Part model, mm, in its own coordinate system. Give positions to 0.01 mm unless a question says otherwise; leave off trailing zeros. Order: outer loops, then holes, each group sorted by start corner. A loop starts at its lowest first (then second) coordinate and runs counter-clockwise, first axis right, second up. Notation, with made-up numbers: (23.25, -37) - (79.25, -37) arc R13 ccw to (79.25, -25) - close; hole circle Ø10 at (84.5, -34.75). An arc over 180 degrees is marked (long way). One line per item, written item: value.
```python
from build123d import *

# Parameters (mm, degrees)
SKETCH1_R           = 83.82
BOSS_EXTRUDE1_DEPTH = 4.826
SKETCH3_R           = 4.445
CUT_EXTRUDE1_DEPTH  = 9.652


with BuildPart() as part:
    # Sketch1 → Boss-Extrude1 (new body, symmetric)
    with BuildSketch(Plane(origin=(0, 0, 0), x_dir=(1, 0, 0), z_dir=(0, 1, 0))):
        Circle(SKETCH1_R)
    extrude(amount=BOSS_EXTRUDE1_DEPTH, both=True)

    # Sketch2 → Cut-Revolve1 (revolve, cut)
    with BuildSketch(Plane.XY):
        with BuildLine():
            Line((0, -4.826), (-19.2970404, -4.826))
            ThreePointArc((-19.2970404, -4.826), (-9.985310315, -2.33207385), (-0.381787908, -1.495209354))
            Line((-0.381787908, -1.495209354), (0, -1.495209354))
            Line((0, -1.495209354), (0, -4.826))
        make_face()
    revolve(axis=Axis((0, -18.327530441, 0), (0, 1, 0)), mode=Mode.SUBTRACT)

    # Sketch3 → Cut-Extrude1 (cut)
    with BuildSketch(Plane(origin=(0, 4.826, 0), x_dir=(1, 0, 0), z_dir=(0, 1, 0))):
        Circle(SKETCH3_R)
    extrude(amount=-CUT_EXTRUDE1_DEPTH, mode=Mode.SUBTRACT)


solid = part.part
```
1) Pin check, flat tips, straight feed: pin 1 (4 mm diameter, centred on y = 4, z = -38.5, fed in from -X); pin 2 (4 mm diameter, centred on x = -56, y = 0.5, fed in from +Z). Stop position of each tip, or through.
Outcome:
pin 1: stops at x = -75.46
pin 2: stops at z = 64.11
2) Cut at C-C, the plane x = 74.5. Give the cut face in (y, z), then the cut area to 3 significant figures.
Outcome:
outline: (-4.83, -38.41) - (4.83, -38.41) - (4.83, 38.41) - (-4.83, 38.41) - close
area: 742 mm^2
3) Drill centre lines: line 1 along X through (y, z) = (1, 0) (3 decimals); line 2 along X through (y, z) = (2.5, -3.5). Where is each one in solid material? Low to high. Write a range as from..to.
Outcome:
line 1: x = -83.82..-4.445, 4.445..83.82
line 2: x = -83.75..-2.74, 2.74..83.75
4) Cut at A-A, the plane y = 0. Give the cut face in (x, z) (3 decimals), then the cut area to 3 significant figures.
Outcome:
outline: circle Ø167.64 at (0, 0); hole circle Ø8.89 at (0, 0)
area: 22,000 mm^2
5) Cut at B-B, the plane z = -34. Give the cut face in (x, y).
Outcome:
outline: (-76.61, -4.83) - (76.61, -4.83) - (76.61, 4.83) - (-76.61, 4.83) - close
6) Mould opens along Z. For faces 1 (the cylindrical face through (-0.96, 1.64, 4.34)), 2 (the flat face through (-1, 4.826, 17)), 3 (the cylindrical face through (-10.912, 0.068, -83.107)) say: released by +Z, released by -Z, zero draft, split by the parting line, or undercut.
Outcome:
face 1: undercut
face 2: zero draft
face 3: split by the parting line
